CAD build for the part. Positions are in the model's coordinates, mm. Face numbers are marked on the shaded views. A direction names the side the tool comes from. Give positions to 0.01 mm unless a question says otherwise; leave off trailing zeros. Loops run counter-clockwise (first coordinate to the right, second up) from the corner with the lowest first, then second, coordinate; pieces in that order, holes last.
Item 1: Which spindle directions (+Z, -Z, +X, -X, +Y, -Y) get a long thin tool onto all of the face, cutting with end or side? Do the marked faces 5 and 6. Say none if no direction does.
Item 2: Probe probe 1 along X at (y, z) = (11, 0); probe 2 along X at (y, z) = (2.5, -3); probe 3 along Z at (x, y) = (-37.5, 44). List the from-to ranges inside material, lowest first.
Item 3: Saw through at C-C on y = 12.5. Give the number of separate pieces and of enclosed holes in the cut face, plus the area to 3 significant figures.
Item 4: Saw through at A-A on z = 0. Give the cut face in (x, y), plus the area to 3 significant figures.
Item 5: Saw through at D-D on y = 54.5. Give the cut face in (x, z) (3 decimals).
Item 6: Drop flat-ended pins along their axis: P1, Ø1.5, axis at y = 44, z = -13.5, coming from the -X side; P2, Ø4, axis at x = -2, z = -8.5, coming from the -Y side; P3, Ø16, axis at x = -38, z = 0, coming from the -Y side; P4, Ø15, axis at x = -38.5, z = -4.5, coming from the +Y side. Give the stop position or say it passes through.
Item 7: Mould opens along X. For the marked faces 1, 2, 3 and 4 say: released by +X, released by -X, zero draft, split by the parting line, or undercut.
Item 8: Saw through at B-B on x = -41.5. Give the cut face in (y, z).
Autodesk Inventor part; units mm, degrees
ref_plane "Work Plane1" through (27, 60, 19) normal (0, -1, 0) x (1, 0, 0)
ref_plane "YZ Plane" through (0, 0, 0) normal (1, 0, 0) x (0, 1, 0)
ref_plane "XZ Plane" through (0, 0, 0) normal (0, 1, 0) x (-1, 0, 0)
sketch "Sketch1" plane through (0, 0, 0) normal (0, 0, 1) x (1, 0, 0)
  arc A0 (36, 0) -> (-36, 0) centre (0, 0) ccw
  arc A1 (27, 0) -> (-27, 0) centre (0, 0) ccw
  line L0 (-36, 0) -> (-27, 0)
  line L1 (27, 0) -> (36, 0)
  dimension "d0" = 72
  dimension "d1" = 54
extrude "Extrusion1" add sketch "Sketch1" along normal mid plane 38
ref_plane "Work Plane1" through (27, 60, 19) normal (0, -1, 0) x (1, 0, 0)
sketch "Sketch2" plane through (27, 60, 19) normal (0, -1, 0) x (1, 0, 0)
  line L0 (11, -19) -> (-65, -19) construction
  line L1 (11, -7) -> (-65, -7)
  line L2 (-65, -31) -> (11, -31)
  arc A0 (11, -31) -> (11, -7) centre (11, -19) ccw
  arc A1 (-65, -7) -> (-65, -31) centre (-65, -19) ccw
  line L3 (0, -38) -> (-54, -38) construction
  line L4 (9, 0) -> (9, -38) construction
  point P0 (-27, -19)
  point P1 (-27, -19)
  dimension "d5" = 76
  dimension "d6" = 12
extrude "Extrusion2" add sketch "Sketch2" along normal up to surface (60 mm away)
sketch "Sketch3" plane through (0, 0, 0) normal (0, 0, 1) x (1, 0, 0)
  arc A0 (27, 0) -> (-27, 0) centre (0, 0) ccw
  line L0 (27, 0) -> (-27, 0)
extrude "Extrusion3" cut sketch "Sketch3" along normal through all both and the other way through all
sketch "Sketch4" plane through (0, 0, 0) normal (0, 0, 1) x (1, 0, 0)
  line L0 (38, 60) -> (-38, 60)
  line L1 (-50, 60) -> (-38, 60)
  line L2 (-50, 60) -> (-50, 0)
  line L3 (-50, 40) -> (-25, 60)
  line L4 (-50, 60) -> (-50, 40)
  point P0 (0, 0)
  dimension "d11" = 25
  dimension "d12" = 20
extrude "Extrusion4" cut sketch "Sketch4" along normal through all both and the other way through all
mirror "Mirror1" about plane through (0, 0, 0) normal (1, 0, 0) of "Extrusion4"
fillet "Fillet1" radius 3 2 edges at (0, 36, -12) (0, 36, 12)
fillet "Fillet2" radius 10 2 edges at (-25, 60, 0) (25, 60, 0)
sketch "Sketch5" plane through (-36, 0, 19) normal (0, -1, 0) x (1, 0, 0)
  arc A0 (-2.8, -7.0267) -> (-2.8, -30.9733) centre (-2, -19) ccw
  point P0 (36, -19)
hole "Hole1" at (-38, 0, 0) direction (0, 1, 0) diameter 10 end through all
sketch "Sketch6" plane through (27, 0, -19) normal (0, -1, 0) x (1, 0, 0)
  arc A0 (11.8, 7.0267) -> (11.8, 30.9733) centre (11, 19) ccw
  point P0 (-27, 19)
hole "Hole2" at (38, 0, 0) direction (0, 1, 0) diameter 10 end through all
sketch "Sketch7" plane through (27, 60, 19) normal (0, 1, 0) x (1, 0, 0)
  circle A0 centre (-65, 19) radius 5
  circle A1 centre (11, 19) radius 5
  circle A2 centre (-65, 19) radius 5
  point P0 (-27, 19)
hole "Hole3" at (-38, 60, 0) at (38, 60, 0) direction (0, -1, 0) diameter 10 end through all counterbore diameter 19 counterbore depth 25
equation "\"d22\" = Thickness"
equation "\"BendRadius\" = Thickness"
equation "\"BendReliefWidth\" = Thickness"
equation "\"BendReliefDepth\" = 0.5 * Thickness"
equation "\"CornerReliefSize\" = 4 * Thickness"
equation "\"MinimumRemnant\" = 2 * Thickness"
equation "\"TransitionRadius\" = BendRadius"
equation "\"JacobiRadiusSize\" = BendRadius"
equation "\"GapSize\" = Thickness"
properties part number "Part4 CONNECTING CAP" material "Stainless Steel"
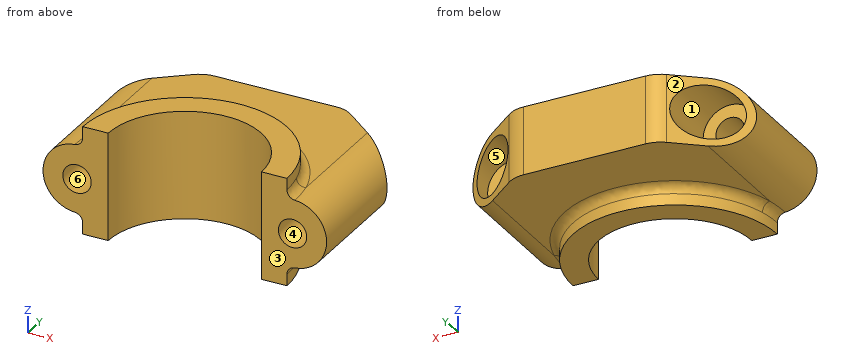
Results below:
1. face 5: +Y
1. face 6: +Y, -Y
2. probe 1: x = -50 to -43, -33 to -24.66, 24.66 to 33, 43 to 50
2. probe 2: x = -49.62 to -42, -34 to -26.88, 26.88 to 34, 42 to 49.62
2. probe 3: z = -12 to -9.49, 9.49 to 12
3. separate pieces: 2
3. enclosed holes: 2
3. area: 1,250 mm2
4. outline: (-50, 0) - (-43, 0) - (-43, 35) - (-47.5, 35) - (-47.5, 42) - (-50, 40) - close; (-33, 0) - (-27, 0) arc R27 cw to (27, 0) - (33, 0) - (33, 35) - (28.5, 35) - (28.5, 57.2) - (27.74, 57.81) arc R10 ccw to (21.49, 60) - (-21.49, 60) arc R10 ccw to (-27.74, 57.81) - (-28.5, 57.2) - (-28.5, 35) - (-33, 35) - close; (43, 0) - (50, 0) - (50, 40) - (47.5, 42) - (47.5, 35) - (43, 35) - close
4. area: 3,100 mm2
5. outline: (-31.875, -12) - (31.875, -12) - (31.875, -7.262) arc R9.5 cw to (31.875, 7.262) - (31.875, 12) - (-31.875, 12) - (-31.875, 7.262) arc R9.5 cw to (-31.875, -7.262) - close
6. P1: passes through
6. P2: stops at y = 26.7
6. P3: stops at y = 0
6. P4: stops at y = 54.91
7. face 1: undercut
7. face 2: released by -X
7. face 3: zero draft
7. face 4: undercut
8. outline: (0, -11.48) - (46.8, -11.48) - (46.8, -8.83) - (35, -8.83) - (35, -3.57) - (0, -3.57) - close; (0, 3.57) - (35, 3.57) - (35, 8.83) - (46.8, 8.83) - (46.8, 11.48) - (0, 11.48) - close
